Read the model definition and answer for the solid it produces. Units are mm, in the model's axes. Face numbers are marked on the shaded views. A direction names the side the tool comes from. Round coordinates to 2 decimals unless told otherwise and drop trailing zeros. Order: outer loops, then holes, each group sorted by start corner. A loop starts at its lowest first (then second) coordinate and runs counter-clockwise, first axis right, second up. Notation, with made-up numbers: (15, 75.5) - (48, 75.5) arc R16 cw to (48, 93.5) - close; hole circle Ø11 at (38.5, -22.5). An arc over 180 degrees is marked (long way). One line per question, with ' | ' between items. Start each with the question number.
1) Straight lines are drawn through the part: line 1 (Z direction, x = -11.5, y = 2); line 2 (Z direction, x = 14, y = -1.5); line 3 (X direction, y = 3.5, z = 15.5). For each, find the intervals that lie inside material, in ascending order. Write a range as from..to.
2) The part is cut by section C-C, the plane z = 4.5. Give the vertices of the cut face in (x, y).
3) For the marked faces 1, 2 and 3, determine the directions among +Z, -Z, +X, -X, +Y, -Y from which every point of the face is accessible in a straight line to the end or side of a thin tool.
4) Flat-ended cylindrical pins translate along their axes: pin 1 (8 mm diameter, centred on x = 10, z = 16.5, fed in from -Y); pin 2 (3 mm diameter, centred on y = 11.5, z = -9.5, fed in from -X); pin 3 (6 mm diameter, centred on x = -8, z = 7.5, fed in from +Y). Find the tip coordinate at first contact, or state that the pin passes through.
5) The mould has two halves that part along Y. Classify the marked faces 4 and 5: pulls with the +Y half, pulls with the -Y half, needs draft (parallel to the pull), parting line crosses it, or undercut.
6) The part is cut by section D-D, the plane z = 9. Give the vertices of the cut face in (x, y).
from build123d import *

# Parameters (mm, degrees)
F2_SIZE = 2.54
F3_R    = 3.175


with BuildPart() as f1:
    # F0 (on Front) → F1 (revolve)
    with BuildSketch(Plane.XZ):
        with BuildLine():
            Line((12.6746, 20.479507), (0, 20.479507))
            Line((0, 20.479507), (0, -14.699493))
            Line((0, -14.699493), (30.1625, -14.699493))
            Line((30.1625, -14.699493), (30.1625, -10.889493))
            Line((30.1625, -10.889493), (19.05, -4.920493))
            Line((19.05, -4.920493), (14.2621, -4.920493))
            ThreePointArc((14.2621, -4.920493), (13.139568, -4.455525), (12.6746, -3.332993))
            Line((12.6746, -3.332993), (12.6746, 6.636507))
            Line((12.6746, 6.636507), (12.6746, 6.638998))
            ThreePointArc((12.6746, 6.638998), (11.609965, 7.133359), (11.176, 8.224007))
            Line((11.176, 8.224007), (11.176, 13.050007))
            ThreePointArc((11.176, 13.050007), (11.609965, 14.140656), (12.6746, 14.635016))
            Line((12.6746, 14.635016), (12.6746, 14.637507))
            Line((12.6746, 14.637507), (12.6746, 20.479507))
        make_face()
    revolve(axis=Axis((0, 0, 2.082966), (0, 0, -1)))

    # F2
    f2_edges = [f1.edges().sort_by_distance(p)[0] for p in [
        (-12.6746, 0, 20.479507),
    ]]
    chamfer(f2_edges, length=F2_SIZE)

    # F3
    f3_edges = [f1.edges().sort_by_distance(p)[0] for p in [
        (-30.1625, 0, -14.699493),
    ]]
    fillet(f3_edges, radius=F3_R)


solid = f1.part
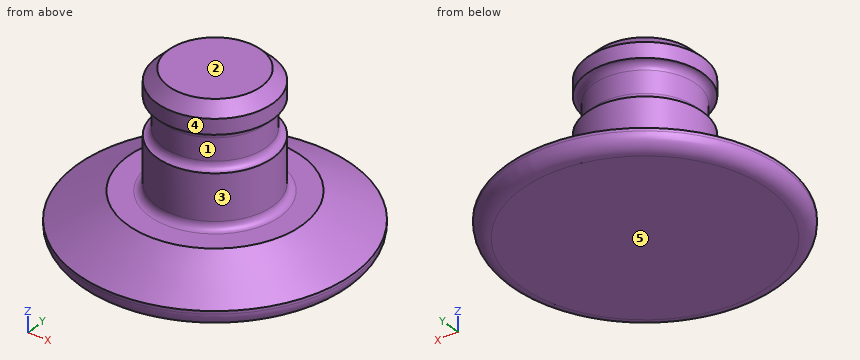
Values:
1) line 1: z = -14.7..7.07, 14.2..18.94 | line 2: z = -14.7..-4.91 | line 3: x = -12.18..12.18
2) outline: circle Ø25.35 at (0, 0)
3) face 1: none | face 2: +Z, +X, -X, +Y, -Y | face 3: +Z
4) pin 1: stops at y = -11.16 | pin 2: stops at x = -28.11 | pin 3: stops at y = 11.59
5) face 4: parting line crosses it | face 5: needs draft
6) outline: circle Ø22.35 at (0, 0)
